Verification items for the finished model (mm, model axes). A direction names the side the tool comes from. Give positions to 0.01 mm unless a question says otherwise; leave off trailing zeros. Loops run counter-clockwise (first coordinate to the right, second up) from the corner with the lowest first, then second, coordinate; pieces in that order, holes last. Notation, with made-up numbers: M 42.25,81.5 L 57.25,81.5 A35 ccw 57.25,120.5 Z; hole C 68,7 d7. An arc over 180 degrees is marked long. Write each question's results on one line, items separated by ' | '. Start each with the question number.
```python
from build123d import *

# Parameters (mm, degrees)
SKETCH3_R                     = 3.25
SKETCH3_R_2                   = 1.5
BOSS_EXTRUDE2_DEPTH           = 11.4
BOSS_EXTRUDE2_TAPER           = 1
BOSS_EXTRUDE2_OTHER_WAY_DEPTH = 1


with BuildPart() as part:
    # Sketch2 → Revolve2 (revolve)
    with BuildSketch(Plane(origin=(0, 0, 0), x_dir=(0, 0, -1), z_dir=(1, 0, 0))):
        Polygon((-2.05, 3.25), (5.45, 3.25), (5.45, 4.25), (2.05, 4.25), (2.05, 7.85), (5.45, 7.85), (5.45, 8.85), (2.95, 8.85), (2.95, 10.45), (-2.95, 10.45), (-2.95, 8.85), (-5.45, 8.85), (-5.45, 7.85), (-2.05, 7.85), align=None)
    revolve(axis=Axis((0, 0, 8.833851455), (0, 0, -1)))

    # Sketch3 → Boss-Extrude2 (add)
    with BuildSketch(Plane.XY.offset(2.05)):
        Circle(SKETCH3_R)
        Circle(SKETCH3_R_2, mode=Mode.SUBTRACT)
    extrude(amount=BOSS_EXTRUDE2_DEPTH, taper=BOSS_EXTRUDE2_TAPER)

    # Sketch3 → Boss-Extrude2 other way (add)
    with BuildSketch(Plane.XY.offset(2.05)):
        Circle(SKETCH3_R)
        Circle(SKETCH3_R_2, mode=Mode.SUBTRACT)
    extrude(amount=-BOSS_EXTRUDE2_OTHER_WAY_DEPTH)


solid = part.part
```
1. Release check for a two-part mould opening along X. For faces 1 (the face through (0.7, 1.5, 1.05)), 2 (the face through (2.66, 8.44, 4.22)), 3 (the face through (1.31, -1.31, 13.45)) record: released by +X, released by -X, zero draft, split by the parting line, or undercut.
2. Section check D-D, the plane z = 4.5. Record the boundary of the cut face in (x, y), plus the area to 3 significant figures.
3. Thickness scan on probe 1 along X at (y, z) = (0, -2.9); probe 2 along Y at (x, z) = (1.75, -4); probe 3 along Y at (x, z) = (-2, -2.75). Record the ranges inside material, lowest first.
4. Depth check by flat-ended pin: pin 1 Ø5.5 at (x, y) = (-3, -2.5) entering from +Z; pin 2 Ø3 at (x, y) = (-8, 5) entering from +Z; pin 3 Ø2 at (x, z) = (2.5, -2) entering from +Y; pin 4 Ø4 at (x, z) = (-6, 6.5) entering from +Y. Enter the tip coordinate at first touch or a pass-through.
5. Set-up check for faces 4 (the face through (5.305, -5.786, 3.726)), 5 (the face through (-3.4, -3.4, -2.05)), 6 (the face through (-1.5, 0.07, 1.56)): record each of +Z, -Z, +X, -X, +Y, -Y from which the full face is reachable in a straight line by a thin tool's end or side.
6. Section check A-A, the plane z = -0.75. Record the boundary of the cut face in (x, y).
7. Section check B-B, the plane x = 6.25. Record the boundary of the cut face in (y, z).
8. Section check C-C, the plane y = -3.75. Record the boundary of the cut face in (x, z), plus the area to 3 significant figures.
Filled sheet:
1) face 1: undercut | face 2: split by the parting line | face 3: zero draft
2) outline: C 0,0 d17.7; C 0,0 d6.41; hole C 0,0 d15.7; hole C 0,0 d3.09 | area: 77.3 mm2
3) probe 1: -10.45 to -7.85, -4.25 to -3.25, 3.25 to 4.25, 7.85 to 10.45 | probe 2: -8.68 to -7.65, -3.87 to -2.74, 2.74 to 3.87, 7.65 to 8.68 | probe 3: -10.26 to -7.59, -3.75 to -2.56, 2.56 to 3.75, 7.59 to 10.26
4) pin 1: z = 13.45 | pin 2: z = 5.45 | pin 3: y = 10.34 | pin 4: y = 7.74
5) face 4: +Z | face 5: -Z | face 6: +Z, -Z
6) outline: C 0,0 d20.9; hole C 0,0 d6.5
7) outline: M -8.37,-2.95 L -6.27,-2.95 L -6.27,-5.45 L -4.75,-5.45 L -4.75,-2.05 L 4.75,-2.05 L 4.75,-5.45 L 6.27,-5.45 L 6.27,-2.95 L 8.37,-2.95 L 8.37,2.95 L 6.27,2.95 L 6.27,5.45 L 4.75,5.45 L 4.75,2.05 L -4.75,2.05 L -4.75,5.45 L -6.27,5.45 L -6.27,2.95 L -8.37,2.95 Z
8) outline: M -9.75,-2.95 L -8.02,-2.95 L -8.02,-5.45 L -6.9,-5.45 L -6.9,-2.05 L -2,-2.05 L -2,-5.45 L 2,-5.45 L 2,-2.05 L 6.9,-2.05 L 6.9,-5.45 L 8.02,-5.45 L 8.02,-2.95 L 9.75,-2.95 L 9.75,2.95 L 8.02,2.95 L 8.02,5.45 L 6.9,5.45 L 6.9,2.05 L -6.9,2.05 L -6.9,5.45 L -8.02,5.45 L -8.02,2.95 L -9.75,2.95 Z | area: 115 mm2
